Verification items for the finished model (mm, model axes). Face numbers are marked on the shaded views. A direction names the side the tool comes from. Give positions to 0.01 mm unless a question says otherwise; leave off trailing zeros. Loops run counter-clockwise (first coordinate to the right, second up) from the corner with the lowest first, then second, coordinate; pieces in that order, holes last. Notation, with made-up numbers: (-32.5, 88.25) - (-7.5, 88.25) arc R17 ccw to (-7.5, 105.25) - close; hole circle Ø4 at (-36.5, 20.25). An arc over 180 degrees is marked (long way). One line per item, written item: value. Start each with the question number.
1. Scan lines: L1, parallel to Z at x = -1.5, y = -12; L2, parallel to Y at x = 0, z = 5. Record each from-to range of solid material in increasing order. Write a range as [from, to].
2. Sectioned sample at C-C (y = -9). Record the cut outline in (x, z) (3 decimals).
3. Sectioned sample at A-A (x = 101.6). Record the cut outline in (y, z).
4. Gauge pin test, flat ends, axial feed: pin 1 (3 mm diameter, centred on y = 3, z = 28, fed in from -X) (3 decimals); pin 2 (1.9 mm diameter, centred on y = 2, z = 3, fed in from +X); pin 3 (3 mm diameter, centred on x = 32, z = 23, fed in from +Y). Record the tip position at first contact, or that the pin passes through.
5. Access from +Z, -Z, +X, -X, +Y, -Y to the whole of each face (thin tool, end or side, straight path). Record for the marked faces 1, 2, 3, 4 and 5.
6. Mould release check, pull along Z, two halves, no side actions. Record for the marked faces 6, 7 and 8: pulls with the +Z half, pulls with the -Z half, needs draft (parallel to the pull), parting line crosses it, or undercut.
7. Sectioned sample at D-D (y = 0). Count the separate pieces of the cut face and the enclosed holes in it, plus the area to 3 significant figures.
8. Sectioned sample at B-B (z = 4.5). Record the cut outline in (x, y).
from build123d import *

# Parameters (mm, degrees)
BOSS_EXTRUDE1_DEPTH     = 38.1
CUT_EXTRUDE1_START      = 6.35
CUT_EXTRUDE1_DEPTH      = 6.35
CUT_EXTRUDE2_DEPTH      = 97.186429746
CUT_EXTRUDE2_DEPTH_BACK = 97.186429746
SKETCH3_R               = 6.35
BOSS_EXTRUDE2_START     = 6.35
SKETCH6_R               = 19.05
BOSS_EXTRUDE2_DEPTH     = 6.35
SKETCH7_R               = 12.7
CUT_EXTRUDE5_DEPTH      = 127.203753906


with BuildPart() as part:
    # Sketch1 → Boss-Extrude1 (new body)
    with BuildSketch(Plane.XY):
        with BuildLine():
            Line((0, 12.7), (87.400968343, 12.7))
            Line((87.400968343, 12.7), (87.400968343, -12.7))
            Line((87.400968343, -12.7), (0, -12.7))
            ThreePointArc((0, -12.7), (-12.7, 0), (0, 12.7))
        make_face()
    extrude(amount=BOSS_EXTRUDE1_DEPTH)

    # Sketch2 → Cut-Extrude1 (cut)
    with BuildSketch(Plane.XY.offset(CUT_EXTRUDE1_START)):
        with BuildLine():
            Line((0, -19.685), (19.685, -19.685))
            Line((19.685, -19.685), (19.685, 19.685))
            Line((19.685, 19.685), (0, 19.685))
            ThreePointArc((0, 19.685), (-19.685, 0), (0, -19.685))
        make_face()
    cut_extrude1 = extrude(amount=CUT_EXTRUDE1_DEPTH, mode=Mode.SUBTRACT)

    # Mirror1: Cut-Extrude1 across plane
    add(cut_extrude1.mirror(Plane(origin=(0, 0, 19.05), x_dir=(1, 0, 0), z_dir=(0, 0, -1))), mode=Mode.SUBTRACT)

    # Sketch3 → Cut-Extrude2 (cut, two sides: drawn at the far end of the back side and taken through both)
    with BuildSketch(Plane.XY.offset(38.1).offset(-CUT_EXTRUDE2_DEPTH_BACK)):
        Circle(SKETCH3_R)
    extrude(amount=CUT_EXTRUDE2_DEPTH + CUT_EXTRUDE2_DEPTH_BACK, mode=Mode.SUBTRACT)

    # Sketch6 → Boss-Extrude2 (add)
    with BuildSketch(Plane(origin=(0, 0, 19.05), x_dir=(-1, 0, 0), z_dir=(0, 0, -1)).offset(BOSS_EXTRUDE2_START)):
        with Locations((-101.6, 0)):
            Circle(SKETCH6_R)
    boss_extrude2 = extrude(amount=BOSS_EXTRUDE2_DEPTH)

    # Sketch7 → Cut-Extrude5 (cut, symmetric)
    with BuildSketch(Plane(origin=(0, 0, 6.35), x_dir=(-1, 0, 0), z_dir=(0, 0, -1))):
        with Locations((-101.6, 0)):
            Circle(SKETCH7_R)
    cut_extrude5 = extrude(amount=CUT_EXTRUDE5_DEPTH, both=True, mode=Mode.SUBTRACT)

    # Mirror3: Boss-Extrude2, Cut-Extrude5 across plane
    add(boss_extrude2.mirror(Plane(origin=(0, 0, 19.05), x_dir=(1, 0, 0), z_dir=(0, 0, -1))))
    add(cut_extrude5.mirror(Plane(origin=(0, 0, 19.05), x_dir=(1, 0, 0), z_dir=(0, 0, -1))), mode=Mode.SUBTRACT)


solid = part.part
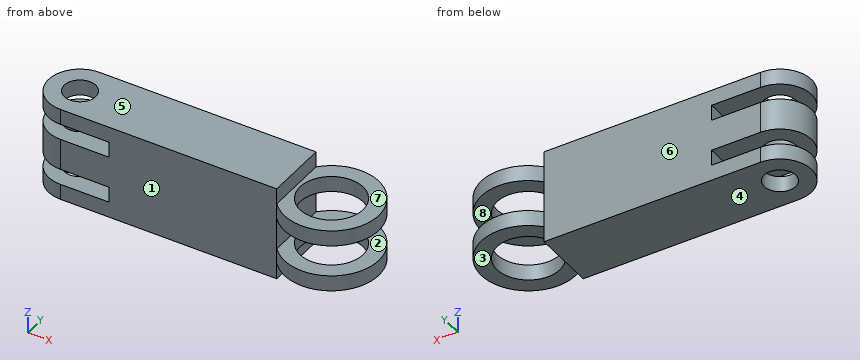
Results are:
1. L1: z = [0, 6.35], [12.7, 25.4], [31.75, 38.1]
1. L2: y = [-12.7, -6.35], [6.35, 12.7]
2. outline: (-8.96, 0) - (87.401, 0) - (87.401, 6.35) - (92.64, 6.35) - (92.64, 12.7) - (87.401, 12.7) - (87.401, 25.4) - (92.64, 25.4) - (92.64, 31.75) - (87.401, 31.75) - (87.401, 38.1) - (-8.96, 38.1) - (-8.96, 31.75) - (19.685, 31.75) - (19.685, 25.4) - (-8.96, 25.4) - (-8.96, 12.7) - (19.685, 12.7) - (19.685, 6.35) - (-8.96, 6.35) - close; (110.56, 6.35) - (118.39, 6.35) - (118.39, 12.7) - (110.56, 12.7) - close; (110.56, 25.4) - (118.39, 25.4) - (118.39, 31.75) - (110.56, 31.75) - close
3. outline: (-19.05, 6.35) - (-12.7, 6.35) - (-12.7, 12.7) - (-19.05, 12.7) - close; (-19.05, 25.4) - (-12.7, 25.4) - (-12.7, 31.75) - (-19.05, 31.75) - close; (12.7, 6.35) - (19.05, 6.35) - (19.05, 12.7) - (12.7, 12.7) - close; (12.7, 25.4) - (19.05, 25.4) - (19.05, 31.75) - (12.7, 31.75) - close
4. pin 1: stops at x = 19.685
4. pin 2: stops at x = 87.4
4. pin 3: stops at y = 12.7
5. face 1: +Z, -Z, -X, -Y
5. face 2: +X, +Y, -Y
5. face 3: -Z, +X, +Y, -Y
5. face 4: -Z, +X, -X, +Y, -Y
5. face 5: +Z, +X, -X, +Y, -Y
6. face 6: needs draft
6. face 7: pulls with the +Z half
6. face 8: undercut
7. separate pieces: 6
7. enclosed holes: 0
7. area: 3,180 mm^2
8. outline: (0, -12.7) - (87.4, -12.7) - (87.4, 12.7) - (0, 12.7) arc R12.7 ccw to start; hole circle Ø12.7 at (0, 0)
